Model file for the job. Use its own axes, mm. Face numbers are marked on the shaded views. Round coordinates to 2 decimals unless told otherwise and drop trailing zeros. Order: outer loops, then holes, each group sorted by start corner. A loop starts at its lowest first (then second) coordinate and runs counter-clockwise, first axis right, second up. Notation, with made-up numbers: (-32, 8.5) -> (21, 8.5) arc R22 ccw to (21, 47.5) -> close; hole circle Ø5 at (57.5, -28). An arc over 180 degrees is marked (long way). Put each result on its own line as item: value. Start each with the question number.
Q1. Flat gauge pins, fed straight in: P1, Ø2, axis at x = -13.5, z = -15, coming from the -Y side; P2, Ø4, axis at y = 17, z = -27, coming from the -X side; P3, Ø10, axis at x = -5.5, y = -0.5, coming from the +Z side. Where does each tip first touch, or does it go through?
Q2. Cut at B-B, the plane x = -24. List the corners of the cut face in (y, z).
Q3. Cut at A-A, the plane y = 0. List the corners of the cut face in (x, z).
Q4. Cut at C-C, the plane y = 19. State how many separate pieces and enclosed holes the cut face has, and give its area (3 significant figures).
Q5. Pull direction Y, two halves, no side cores. Call the marked faces 1, 2, 3 and 4: released by +Y, released by -Y, zero draft, split by the parting line, or undercut.
Q6. Probe L1, parallel to Y at x = -11.15, z = 0; L2, parallel to X at y = 0, z = -26.5; L3, parallel to Z at x = 11, y = 26. List the from-to ranges inside material, lowest first.
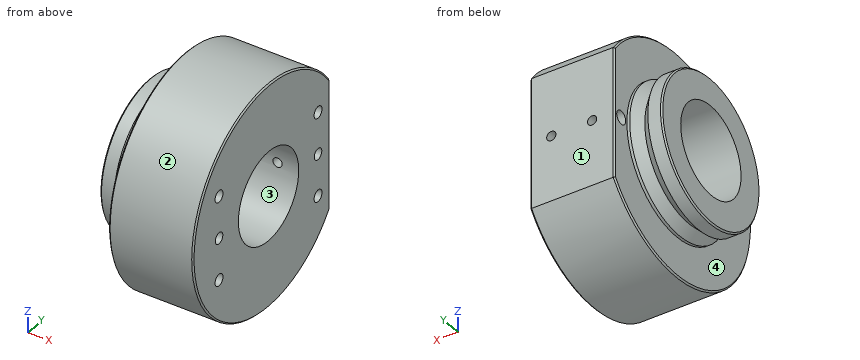
from build123d import *

# Parameters (mm, degrees)
CHAMFER1_SIZE                   = 0.5
SKETCH3_W                       = 30.914832272
SKETCH3_H                       = 82.011072724
CUT_EXTRUDE2_DEPTH              = 7.5
CHAMFER2_SIZE                   = 0.5
F_3_16_0_1875_DOWEL_HOLE1_D     = 4.7625
F_3_16_0_1875_DOWEL_HOLE1_DEPTH = 5.5
F_3_16_0_1875_DOWEL_HOLE1_TIP   = 1.430799349
M5X0_8_TAPPED_HOLE1_D           = 4.2
M5X0_8_TAPPED_HOLE1_DEPTH       = 12.4
M5X0_8_TAPPED_HOLE1_TIP         = 1.2618073
F_4_0MM_DOWEL_HOLE1_D           = 4
F_4_0MM_DOWEL_HOLE1_DEPTH       = 5.2
F_4_0MM_DOWEL_HOLE1_TIP         = 1.201721238
M4X0_7_TAPPED_HOLE1_REACH       = 89.275
M4X0_7_TAPPED_HOLE1_BORE_R      = 1.65


with BuildPart() as part:
    # Sketch1 → Revolve1 (revolve)
    with BuildSketch(Plane.XY, mode=Mode.PRIVATE) as revolve1_sk:
        Polygon((-27.58192079, 26), (-22.58192079, 26), (-19.361510024, 22.779589234), (-16.141099258, 26), (-15.141099258, 26), (-15.141099258, 40), (14.858900742, 40), (14.858900742, 16), (-27.58192079, 16), align=None)
    revolve(revolve1_sk.sketch.rotate(Axis((-39.738562092, 0, 0), (1, 0, 0)), 90), axis=Axis((-39.738562092, 0, 0), (1, 0, 0)))

    # Chamfer1
    chamfer1_edges = [part.edges().sort_by_distance(p)[0] for p in [
        (-27.58192079, 0, -26),
        (14.858900742, 0, -40),
        (-15.141099258, 0, -40),
    ]]
    chamfer(chamfer1_edges, length=CHAMFER1_SIZE)

    # Sketch3 → Cut-Extrude2 (cut)
    with BuildSketch(Plane(origin=(0, 40, 0), x_dir=(1, 0, 0), z_dir=(0, 1, 0))):
        with Locations((-0.069893973, 0.224952002)):
            Rectangle(SKETCH3_W, SKETCH3_H)
    extrude(amount=-CUT_EXTRUDE2_DEPTH, mode=Mode.SUBTRACT)

    # Chamfer2
    chamfer2_edges = [part.edges().sort_by_distance(p)[0] for p in [
        (14.858900742, 32.5, 0),
        (-15.141099258, 32.5, 0),
    ]]
    chamfer(chamfer2_edges, length=CHAMFER2_SIZE)

    # 3/16 (0.1875) Dowel Hole1
    with Locations(Plane.ZY.offset(15.141099258)):
        with Locations((0, 29)):
            Hole(F_3_16_0_1875_DOWEL_HOLE1_D / 2, depth=F_3_16_0_1875_DOWEL_HOLE1_DEPTH)
            with Locations((0, 0, -(F_3_16_0_1875_DOWEL_HOLE1_DEPTH + F_3_16_0_1875_DOWEL_HOLE1_TIP / 2))):  # 118° drill point
                Cone(0, F_3_16_0_1875_DOWEL_HOLE1_D / 2, F_3_16_0_1875_DOWEL_HOLE1_TIP, mode=Mode.SUBTRACT)

    # M5x0.8 Tapped Hole1
    with Locations(Plane(origin=(14.858900742, 0, 0), x_dir=(0, 0, -1), z_dir=(1, 0, 0))):
        with Locations((-15, 26.25), (15, 26.25), (-15, -26.25), (15, -26.25)):
            Hole(M5X0_8_TAPPED_HOLE1_D / 2, depth=M5X0_8_TAPPED_HOLE1_DEPTH)
            with Locations((0, 0, -(M5X0_8_TAPPED_HOLE1_DEPTH + M5X0_8_TAPPED_HOLE1_TIP / 2))):  # 118° drill point
                Cone(0, M5X0_8_TAPPED_HOLE1_D / 2, M5X0_8_TAPPED_HOLE1_TIP, mode=Mode.SUBTRACT)

    # Ø4.0mm Dowel Hole1
    with Locations(Plane(origin=(14.858900742, 0, 0), x_dir=(0, 0, -1), z_dir=(1, 0, 0))):
        with Locations((0, 26.25), (0, -26.25)):
            Hole(F_4_0MM_DOWEL_HOLE1_D / 2, depth=F_4_0MM_DOWEL_HOLE1_DEPTH)
            with Locations((0, 0, -(F_4_0MM_DOWEL_HOLE1_DEPTH + F_4_0MM_DOWEL_HOLE1_TIP / 2))):  # 118° drill point
                Cone(0, F_4_0MM_DOWEL_HOLE1_D / 2, F_4_0MM_DOWEL_HOLE1_TIP, mode=Mode.SUBTRACT)

    # M4x0.7 Tapped Hole1 bore → M4x0.7 Tapped Hole1 (cut, up to next)
    with BuildSketch(Plane(origin=(0, 32.5, 0), x_dir=(1, 0, 0), z_dir=(0, 1, 0)), mode=Mode.PRIVATE) as m4x0_7_tapped_hole1_sk1:
        with Locations((-7.141099258, 0)):
            Circle(M4X0_7_TAPPED_HOLE1_BORE_R)
    m4x0_7_tapped_hole1_tool1 = extrude(m4x0_7_tapped_hole1_sk1.sketch, amount=-M4X0_7_TAPPED_HOLE1_REACH, mode=Mode.PRIVATE) & part.part
    # M4x0.7 Tapped Hole1 bore → M4x0.7 Tapped Hole1 (cut, up to next)
    with BuildSketch(Plane(origin=(0, 32.5, 0), x_dir=(1, 0, 0), z_dir=(0, 1, 0)), mode=Mode.PRIVATE) as m4x0_7_tapped_hole1_sk2:
        with Locations((7.358900742, 0)):
            Circle(M4X0_7_TAPPED_HOLE1_BORE_R)
    m4x0_7_tapped_hole1_tool2 = extrude(m4x0_7_tapped_hole1_sk2.sketch, amount=-M4X0_7_TAPPED_HOLE1_REACH, mode=Mode.PRIVATE) & part.part
    add(m4x0_7_tapped_hole1_tool1.solids().sort_by_distance((-7.141099, 32.5, 0))[0], mode=Mode.SUBTRACT)
    add(m4x0_7_tapped_hole1_tool2.solids().sort_by_distance((7.358901, 32.5, 0))[0], mode=Mode.SUBTRACT)


solid = part.part
Ans:
1. P1: stops at y = -37.47
1. P2: stops at x = -15.14
1. P3: stops at z = 40
2. outline: circle Ø52 at (0, 0); hole circle Ø32 at (0, 0)
3. outline: (-27.58, -25.5) -> (-27.08, -26) -> (-22.58, -26) -> (-19.36, -22.78) -> (-16.14, -26) -> (-15.14, -26) -> (-15.14, -39.5) -> (-14.64, -40) -> (14.36, -40) -> (14.86, -39.5) -> (14.86, -16) -> (-27.58, -16) -> close; (-27.58, 16) -> (14.86, 16) -> (14.86, 39.5) -> (14.36, 40) -> (-14.64, 40) -> (-15.14, 39.5) -> (-15.14, 26) -> (-16.14, 26) -> (-19.36, 22.78) -> (-22.58, 26) -> (-27.08, 26) -> (-27.58, 25.5) -> close
4. separate pieces: 1
4. enclosed holes: 2
4. area: 2,500 mm^2
5. face 1: released by +Y
5. face 2: split by the parting line
5. face 3: undercut
5. face 4: zero draft
6. L1: y = -40 to -16, 16 to 26.62, 31.38 to 32.5
6. L2: x = -15.14 to 14.86
6. L3: z = -30.4 to -17.09, -12.91 to -1.98, 1.98 to 12.91, 17.09 to 30.4
